Study the drawing (mm; zero at the part's minimum x, y, z) and answer. A direction names the side the tool comes from. Coordinates: 2 decimals unless noted, no trailing zeros. Order: outer loops, then holes, each group sorted by start corner. A loop starts at its lowest first (then second) coordinate and runs counter-clockwise, first axis right, second up. Notation, with made-up numbers: (79.5, 5) -> (137.5, 5) arc R26 cw to (137.5, 29) -> close; hole circle Ø4 at (21.5, 76). An arc over 180 degrees is marked (long way). One line per question, with ' | ' between items.
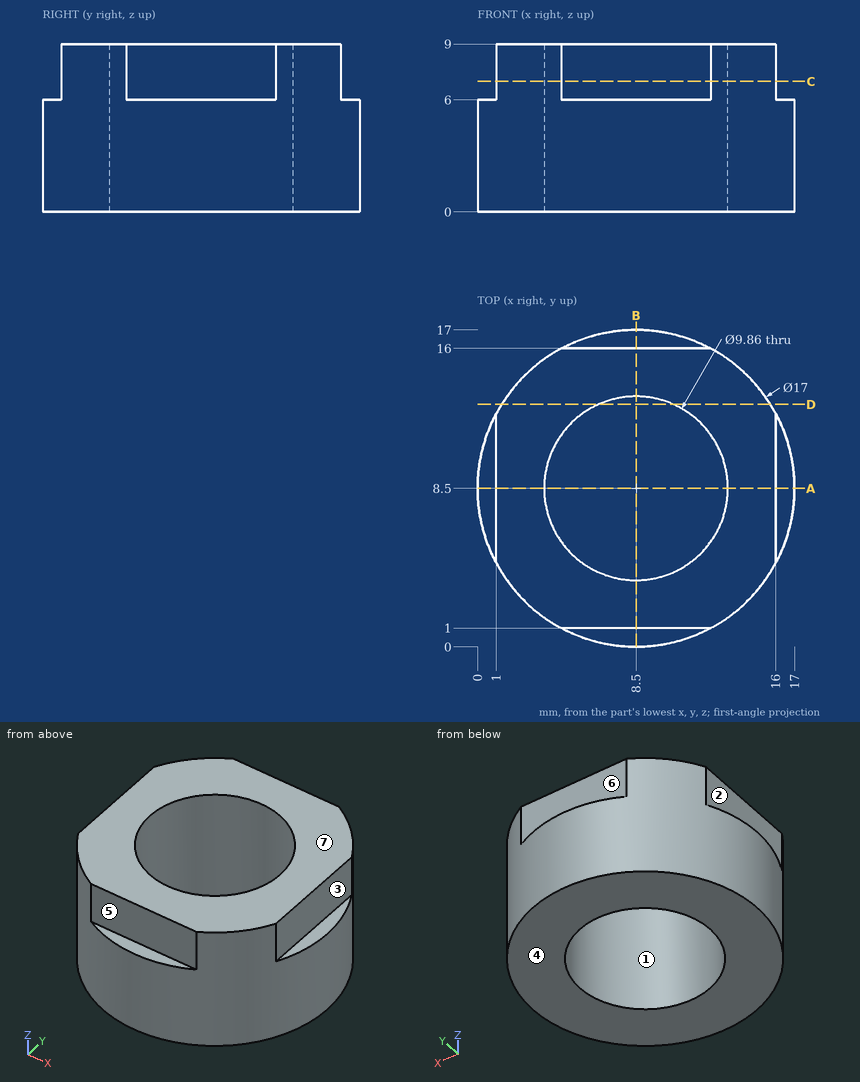
Item 1: Find the intervals of material crossed by L1, parallel to Y at x = 8.5, z = 7.25; L2, parallel to Y at x = 8.5, z = 5.25; L3, parallel to X at y = 9.25, z = 5.75, in increasing order.
Computed values:
L1: y = 1 to 3.57, 13.43 to 16 | L2: y = 0 to 3.57, 13.43 to 17 | L3: x = 0.03 to 3.63, 13.37 to 16.97
Item 2: For the marked faces 5, 6 and 7, determine the directions among +Z, -Z, +X, -X, +Y, -Y from which every point of the face is accessible in a straight line to the end or side of a thin tool.
Computed values:
face 5: +Z, +X, -X, -Y | face 6: +Z, +X, -X, +Y | face 7: +Z, +X, -X, +Y, -Y
Item 3: Section D-D, the plane y = 13 is taken. Give the vertices of the cut face in (x, z).
Computed values:
outline: (1.29, 0) -> (6.49, 0) -> (6.49, 9) -> (1.29, 9) -> close; (10.51, 0) -> (15.71, 0) -> (15.71, 9) -> (10.51, 9) -> close
Item 4: Determine the mould class of the marked faces 1, 2, 3 and 4 for opening direction X: pulls with the +X half, pulls with the -X half, needs draft (parallel to the pull), parting line crosses it, or undercut.
Computed values:
face 1: undercut | face 2: pulls with the -X half | face 3: pulls with the +X half | face 4: needs draft
Item 5: Section C-C, the plane z = 7 is taken. Give the vertices of the cut face in (x, y), plus the area to 3 significant figures.
Computed values:
outline: (1, 4.5) arc R8.5 ccw to (4.5, 1) -> (12.5, 1) arc R8.5 ccw to (16, 4.5) -> (16, 12.5) arc R8.5 ccw to (12.5, 16) -> (4.5, 16) arc R8.5 ccw to (1, 12.5) -> close; hole circle Ø9.86 at (8.5, 8.5) | area: 129 mm^2
Item 6: Section A-A, the plane y = 8.5 is taken. Give the vertices of the cut face in (x, z).
Computed values:
outline: (0, 0) -> (3.57, 0) -> (3.57, 9) -> (1, 9) -> (1, 6) -> (0, 6) -> close; (13.43, 0) -> (17, 0) -> (17, 6) -> (16, 6) -> (16, 9) -> (13.43, 9) -> close
Item 7: Each of these flat-tipped pins is pushed along its axis until it touches: pin 1 Ø3.5 at (y, z) = (9.5, 7.5) entering from -X; pin 2 Ø0.9 at (x, z) = (7, 7.5) entering from -Y; pin 3 Ø1.5 at (y, z) = (10, 7) entering from +X; pin 4 Ø2.5 at (x, z) = (10, 7) entering from +Y. Where does it stop, or does it pass through?
Computed values:
pin 1: stops at x = 0 | pin 2: stops at y = 1 | pin 3: stops at x = 16 | pin 4: stops at y = 16.97
